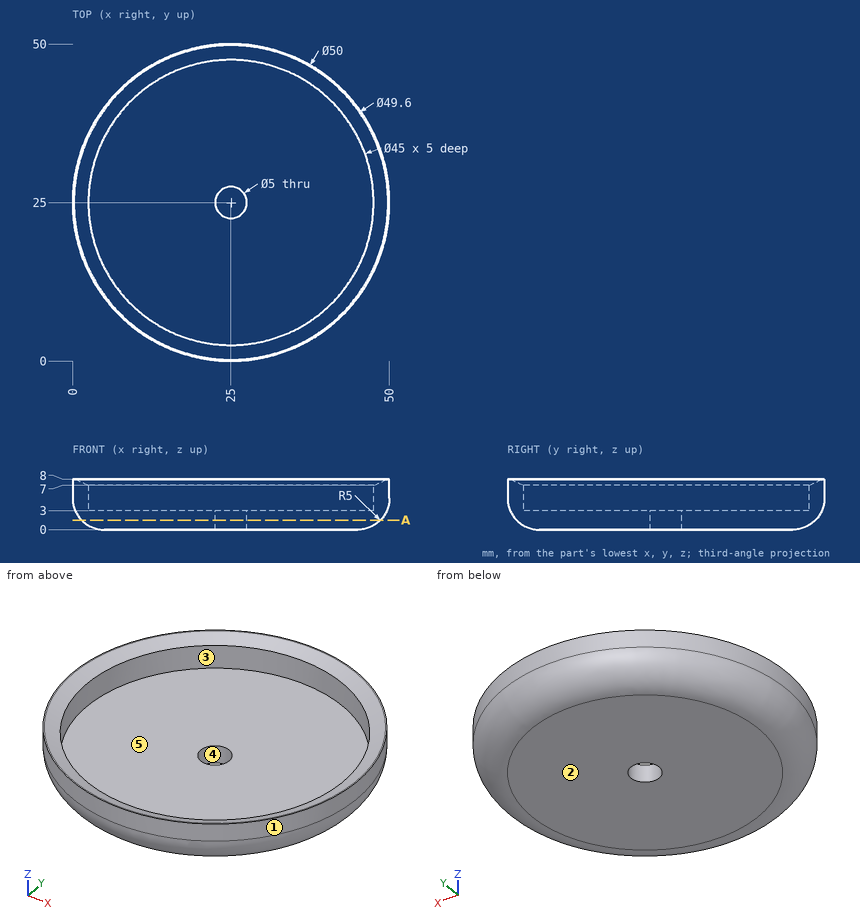
Can you work these out from the drawing? Everything is in mm from the part's minimum corner. A direction names the side the tool comes from. Round coordinates to 2 decimals unless told otherwise and drop trailing zeros. Loops run counter-clockwise (first coordinate to the right, second up) from the corner with the lowest first, then second, coordinate; pieces in that order, holes last. Notation, with made-up numbers: (78, -16) - (94, -16) arc R25 ccw to (94, 2) - close; hole circle Ø4 at (53, 6). An arc over 180 degrees is marked (long way). Write item = value, one per line. Start each with the question number.
(1) If we mould it in two halves opening along X, with no side actions, what happens to the marked faces 1, 2 and 3? For each: released by +X, released by -X, zero draft, split by the parting line, or undercut.
(2) For the marked faces 4 and 5, which set-ups out of +Z, -Z, +X, -X, +Y, -Y let a thin tool reach every point of the face, with its end or its side?
(3) For P1, Ø1.5, axis at y = 37.5, z = 4.5, coming from the -X side; P2, Ø6, axis at x = 16, y = 34.5, coming from the +Z side; P3, Ø3, axis at x = 25, y = 25, coming from the +Z side; P4, Ø4, axis at x = 15, z = 2, coming from the -Y side, each with a flat end and sliding along its axis, tell me the tip position at first contact or that it passes through.
(4) If we section it at A-A (z = 1.5): Please give me the cut outline in (x, y), and give its area (3 significant figures).
(5) If I drill on probe 1 along Y at (x, z) = (25, 5.85); probe 2 along Y at (x, z) = (28.5, 3.5); probe 3 along Z at (x, y) = (40, 28), over which ranges is the centre line in solid material (lowest first)? Write a range as [from, to].
Ans:
q1.face_1 = split by the parting line
q1.face_2 = zero draft
q1.face_3 = undercut
q2.face_4 = +Z, -Z
q2.face_5 = +Z
q3.P1 = 2.95
q3.P2 = 3
q3.P3 = through
q3.P4 = 1.8
q4.outline = circle Ø47.14 at (25, 25); hole circle Ø5 at (25, 25)
q4.area = 1,730 mm²
q5.probe_1 = [0, 2.5], [47.5, 50]
q5.probe_2 = [0.48, 2.77], [47.23, 49.52]
q5.probe_3 = [0, 3]
